```python
from build123d import *

# Parameters (mm, degrees)
SKETCH_1_W          = 148
SKETCH_1_H          = 166
EXTRUDE_1_DEPTH     = 3
SKETCH_2_R          = 2.5
CUT_EXTRUDE_1_DEPTH = 4


with BuildPart() as part:
    # 草图1 → 凸台-拉伸1 (new body)
    with BuildSketch(Plane(origin=(0, 0, 0), x_dir=(1, 0, 0), z_dir=(0, 1, 0))):
        Rectangle(SKETCH_1_W, SKETCH_1_H)
    extrude(amount=EXTRUDE_1_DEPTH)

    # 草图2 → 切除-拉伸1 (cut, through all)
    with BuildSketch(Plane(origin=(0, 3, 0), x_dir=(1, 0, 0), z_dir=(0, 1, 0))):
        with Locations((-58, 51.5)):
            Circle(SKETCH_2_R)
        with Locations((-27.5, 51.5)):
            Circle(SKETCH_2_R)
        with Locations((-27.5, -51.5)):
            Circle(SKETCH_2_R)
        with Locations((-58, -51.5)):
            Circle(SKETCH_2_R)
        with Locations((58, -51.5)):
            Circle(SKETCH_2_R)
        with Locations((27.5, -51.5)):
            Circle(SKETCH_2_R)
        with Locations((27.5, 51.5)):
            Circle(SKETCH_2_R)
        with Locations((58, 51.5)):
            Circle(SKETCH_2_R)
        with Locations((-42.75, 71)):
            Circle(SKETCH_2_R)
        with Locations((-42.75, -71)):
            Circle(SKETCH_2_R)
        with Locations((42.75, -71)):
            Circle(SKETCH_2_R)
        with Locations((42.75, 71)):
            Circle(SKETCH_2_R)
        with Locations((-62, 0)):
            Circle(SKETCH_2_R)
        with Locations((-42.5, -15.25)):
            Circle(SKETCH_2_R)
        with Locations((-42.5, 15.25)):
            Circle(SKETCH_2_R)
        with Locations((42.5, 15.25)):
            Circle(SKETCH_2_R)
        with Locations((42.5, -15.25)):
            Circle(SKETCH_2_R)
        with Locations((62, 0)):
            Circle(SKETCH_2_R)
    extrude(amount=-CUT_EXTRUDE_1_DEPTH, mode=Mode.SUBTRACT)


solid = part.part
```
Verification items for the finished model (mm, model axes). Round coordinates to 2 decimals unless told otherwise and drop trailing zeros. Loops run counter-clockwise (first coordinate to the right, second up) from the corner with the lowest first, then second, coordinate; pieces in that order, holes last. Notation, with made-up numbers: (55, -21.75) -> (91, -21.75) arc R13 ccw to (91, -1.75) -> close; hole circle Ø2 at (50.5, -32). An arc over 180 degrees is marked (long way). Answer as a JSON object with one key per item and string values.
Q1. Section check B-B (x = -27.5). Record the boundary of the cut face in (y, z), then the cut area to 3 significant figures.
Data:
{"outline": "(0, -83) -> (3, -83) -> (3, -54) -> (0, -54) -> close; (0, -49) -> (3, -49) -> (3, 49) -> (0, 49) -> close; (0, 54) -> (3, 54) -> (3, 83) -> (0, 83) -> close", "area": "468 mm2"}
Q2. Section check A-A (z = 51.5). Record the boundary of the cut face in (x, y).
Data:
{"outline": "(-74, 0) -> (-60.5, 0) -> (-60.5, 3) -> (-74, 3) -> close; (-55.5, 0) -> (-30, 0) -> (-30, 3) -> (-55.5, 3) -> close; (-25, 0) -> (25, 0) -> (25, 3) -> (-25, 3) -> close; (30, 0) -> (55.5, 0) -> (55.5, 3) -> (30, 3) -> close; (60.5, 0) -> (74, 0) -> (74, 3) -> (60.5, 3) -> close"}
Q3. Section check D-D (z = -71). Record the boundary of the cut face in (x, y), then the cut area to 3 significant figures.
Data:
{"outline": "(-74, 0) -> (-45.25, 0) -> (-45.25, 3) -> (-74, 3) -> close; (-40.25, 0) -> (40.25, 0) -> (40.25, 3) -> (-40.25, 3) -> close; (45.25, 0) -> (74, 0) -> (74, 3) -> (45.25, 3) -> close", "area": "414 mm2"}
Q4. Draft check along X on faces 1 (the flat face through (-1, 0, -1)), 2 (the cylindrical face through (45.06, 1.52, -70.04)). Enter one of: pulls with the +X half, pulls with the -X half, needs draft (parallel to the pull), parting line crosses it, or undercut.
Data:
{"face 1": "needs draft", "face 2": "undercut"}
Q5. Scan lines: line 1 (X direction, y = 2.35, z = 51.5); line 2 (X direction, y = 1.6, z = 15); line 3 (Z direction, x = -58, y = 1.6). Record each from-to range of solid material in increasing order. Write a range as from..to.
Data:
{"line 1": "x = -74..-60.5, -55.5..-30, -25..25, 30..55.5, 60.5..74", "line 2": "x = -74..-44.99, -40.01..40.01, 44.99..74", "line 3": "z = -83..-54, -49..49, 54..83"}
Q6. Section check C-C (x = -42.5). Record the boundary of the cut face in (y, z).
Data:
{"outline": "(0, -83) -> (3, -83) -> (3, -73.49) -> (0, -73.49) -> close; (0, -68.51) -> (3, -68.51) -> (3, -17.75) -> (0, -17.75) -> close; (0, -12.75) -> (3, -12.75) -> (3, 12.75) -> (0, 12.75) -> close; (0, 17.75) -> (3, 17.75) -> (3, 68.51) -> (0, 68.51) -> close; (0, 73.49) -> (3, 73.49) -> (3, 83) -> (0, 83) -> close"}
